from build123d import *

# Parameters (mm, degrees)
F1_DEPTH  = 33.02
F2_R      = 18.3561977424
F3_DEPTH  = 38.1
F4_R      = 5.2507259391
F5_DEPTH  = 68.58
F7_DEPTH  = 51.054
F8_R      = 4.7656912357
F8_R_2    = 10.9843884843
F8_R_3    = 9.697479166
F8_R_4    = 9.2479292762
F8_R_5    = 8.5292895708
F8_R_6    = 7.1733155085
F8_R_7    = 8.6736896771
F8_R_8    = 5.4464276584
F8_R_9    = 8.102554369
F8_R_10   = 5.3943968671
F8_R_11   = 6.0751011196
F8_R_12   = 5.9571165591
F8_R_13   = 3.4735651016
F9_DEPTH  = 19.05
F11_W     = 74.5131336153
F11_H     = 36.8404686451
F11_W_2   = 35.7296550646
F11_H_2   = 10.0775975734
F11_W_3   = 29.0112560615
F11_H_3   = 10.3829782456
F11_H_4   = 11.6045051254
F12_DEPTH = 4.064
F14_DEPTH = 5.842


with BuildPart() as f1:
    # F0 (on Right) → F1 (new body)
    with BuildSketch(Plane.YZ):
        Polygon((0, 55.1033206284), (-40.2105264366, 34.8491296172), (-40.2105264366, -55.6990355253), (39.6148264408, -55.6990355253), (39.6148264408, 34.8491296172), align=None)
        Polygon((-59.7306484823, 25.0167718862), (-40.2105264366, 34.8491296172), (0, 55.1033206284), (39.6148264408, 34.8491296172), (58.8457670794, 25.0167718862), (53.8931720944, 34.8491296172), (0, 62.4035252784), (-54.703579845, 34.8491296172), align=None)
    extrude(amount=F1_DEPTH)

    # F2 (on face) → F3 (cut)
    with BuildSketch(Plane.YZ.offset(33.02)):
        with Locations((0, 11.9900638238)):
            Circle(F2_R)
    extrude(amount=-F3_DEPTH, mode=Mode.SUBTRACT)

    # F4 (on face) → F5 (join)
    with BuildSketch(Plane.YZ.offset(33.02)):
        with Locations((0, -33.2840159535)):
            Circle(F4_R)
    extrude(amount=F5_DEPTH)

    # F6 (on face) → F7 (join)
    with BuildSketch(Plane(origin=(0, 0, 0), x_dir=(0, -1, 0), z_dir=(-1, 0, 0))):
        Polygon((-53.8931720944, 34.8491296172), (-58.8457670794, 25.0167718862), (-39.6148264408, 34.8491296172), (-39.6148264408, -55.6990355253), (40.2105264366, -55.6990355253), (40.2105264366, 34.8491296172), (59.7306484823, 25.0167718862), (54.703579845, 34.8491296172), (0, 62.4035252784), align=None)
    extrude(amount=F7_DEPTH)

    # F8 (on face) → F9 (cut)
    with BuildSketch(Plane(origin=(0, 39.6148264408, 0), x_dir=(-1, 0, 0), z_dir=(0, 1, 0))):
        with Locations((-19.2792955786, -27.9984436929)):
            Circle(F8_R)
        with Locations((7.5277197175, -25.0198859721)):
            Circle(F8_R_2)
        with Locations((18.2505380362, 0)):
            Circle(F8_R_3)
        with Locations((-18.0878732353, 8.9356740937)):
            Circle(F8_R_4)
        with Locations((-11.5350466222, -11.9142318144)):
            Circle(F8_R_5)
        with Locations((36.7175936699, 15.4885025695)):
            Circle(F8_R_6)
        with Locations((33.7390340865, -20.8499059081)):
            Circle(F8_R_7)
        with Locations((0, 14.2970783636)):
            Circle(F8_R_8)
        with Locations((27.1862093359, -39.3169634044)):
            Circle(F8_R_9)
        with Locations((-15.1093155146, -45.2740825713)):
            Circle(F8_R_10)
        with Locations((6.9320080802, -45.8697937429)):
            Circle(F8_R_11)
        with Locations((42.0789942145, 0)):
            Circle(F8_R_12)
        with Locations((43.2704202831, -37.5298298895)):
            Circle(F8_R_13)
    extrude(amount=-F9_DEPTH, mode=Mode.SUBTRACT)

    # F11 (on face) → F12 (join)
    with BuildSketch(Plane.XZ.offset(40.2105264366)):
        with Locations((-10.0858341902, -18.4202343225)):
            Rectangle(F11_W, F11_H)
        with Locations((-26.1183748953, -26.9155642018)):
            Rectangle(F11_W_2, F11_H_2, mode=Mode.SUBTRACT)
        with Locations((9.9166636355, -27.0682545379)):
            Rectangle(F11_W_3, F11_H_3, mode=Mode.SUBTRACT)
        with Locations((-26.1183748953, -9.9668807816)):
            Rectangle(F11_W_2, F11_H_4, mode=Mode.SUBTRACT)
        with Locations((9.9166636355, -9.9668807816)):
            Rectangle(F11_W_3, F11_H_4, mode=Mode.SUBTRACT)
    extrude(amount=F12_DEPTH)

    # F13 (on face) → F14 (join)
    with BuildSketch(Plane(origin=(-51.054, 0, 0), x_dir=(0, -1, 0), z_dir=(-1, 0, 0))):
        Polygon((3.0381854158, 2.3930334493), (3.0381854158, 23.5505028621), (-15.2847205754, 12.9717681557), align=None)
        Polygon((-8.2609392703, 25.3185906107), (-8.2609392703, 50.7075435822), (-30.248417519, 38.0130670965), align=None)
        Polygon((32.9538357962, -30.5881882396), (1.2176486146, -9.4307204399), (-1.2371623889, -47.4937986583), align=None)
        Polygon((32.310971557, 4.7542667825), (23.8479883086, 24.8538487713), (10.672731325, 7.474899292), align=None)
        Polygon((-20.1708246022, -26.5583209633), (-20.1708246022, -8.5744783342), (-35.7452891767, -17.5663996488), align=None)
        Polygon((20.4449407756, 28.2686487088), (20.4449407756, 48.3682468286), (3.038178198, 38.3184477687), align=None)
        Polygon((24.4587499026, -20.5924118991), (32.9217363772, -0.4928299103), (11.2834945321, -3.2134596258), align=None)
    extrude(amount=F14_DEPTH)


solid = f1.part
Source: CAD feature listing. Evaluate the final solid. Frame: model axes, mm. A direction names the side the tool comes from. Coordinates: 2 decimals unless noted, no trailing zeros. Loops run counter-clockwise (first coordinate to the right, second up) from the corner with the lowest first, then second, coordinate; pieces in that order, holes last. Notation, with made-up numbers: (29, -17.5) -> (52, -17.5) arc R25 cw to (52, 2.5) -> close; hole circle Ø3 at (67.5, -33). An arc over 180 degrees is marked (long way). Answer in a Markdown table with one row per item. Add a question column.
Q1. Section B-B on z = 41. Return the cut outline in (x, y), and give its area (3 significant figures).
Q2. Ray query, line 1 along Y through (x, z) = (-48, 34.5); line 2 along X through (y, z) = (29, -41.5) (3 decimals); line 3 along X through (y, z) = (35, -37.5). Return the intervals inside material, ascending.
Q3. Reachability of faces 1 (the face through (-53.934, -0.007, -28.196)), 2 (the face through (-8, 39.615, -10)), 3 (the face through (-43.983, -42, -27)), 4 (the face through (-54, 20.171, -18)), 5 (the face through (0.7, 30.2, 19.7)) from +Z, -Z, +X, -X, +Y, -Y: full face, straight path, thin tool, end or side. Return the list, or none.
Q4. Section C-C on x = 91.5. Return the cut outline in (y, z).
Q5. Section A-A on y = 24. Give the number of separate pieces and of enclosed holes in the cut face, and give its area (3 significant figures).
Q6. Pull-direction query (Z, two-part tool) for faces 6 (the face through (66.83, -1.14, -38.41)), 7 (the face through (-8.428, 49.365, 29.864)), 8 (the face through (-27, 20.565, -39)); classes: pulls with the +Z half, pulls with the -Z half, needs draft (parallel to the pull), parting line crosses it, or undercut.
Q7. Contact query for flat-ended pins moving along their axis: pin 1 Ø2 at (x, y) = (4.5, 43) entering from +Z; pin 2 Ø1.2 at (y, z) = (-41.5, -23.5) entering from +X; pin 3 Ø2 at (y, z) = (29.5, 5.5) entering from -X; pin 4 Ø4.5 at (x, y) = (15.5, -41.5) entering from -Z. Output: stop coordinate, or through.
Computed values:
| question | item | result |
|---|---|---|
| 1 | outline | (-56.9, -20.44) -> (-51.05, -20.44) -> (-51.05, -42.49) -> (33.02, -42.49) -> (33.02, 41.86) -> (-51.05, 41.86) -> (-51.05, 25.07) -> (-56.9, 25.07) -> (-56.9, 8.26) -> (-51.05, 8.26) -> (-51.05, -7.68) -> (-56.9, -7.68) -> close |
| 1 | area | 7,260 mm^2 |
| 2 | line 1 | y = -54.88 to -40.9, -40.21 to 39.61, 40.3 to 54.07 |
| 2 | line 2 | x = -51.054 to -34.989, -19.383 to -11.152, -2.712 to 11.255, 18.964 to 33.02 |
| 2 | line 3 | x = -51.05 to -46.74, -39.8 to -35.08, -19.29 to 33.02 |
| 3 | face 1 | -X |
| 3 | face 2 | -Z, +X, -X |
| 3 | face 3 | -Y |
| 3 | face 4 | -Z, -X |
| 3 | face 5 | +Y |
| 4 | outline | circle Ø10.5 at (0, -33.28) |
| 5 | separate pieces | 1 |
| 5 | enclosed holes | 13 |
| 5 | area | 6,720 mm^2 |
| 6 | face 6 | parting line crosses it |
| 6 | face 7 | pulls with the -Z half |
| 6 | face 8 | undercut |
| 7 | pin 1 | stops at z = 40.93 |
| 7 | pin 2 | stops at x = 27.17 |
| 7 | pin 3 | stops at x = -51.05 |
| 7 | pin 4 | stops at z = -55.7 |
